from build123d import *

# Parameters (mm, degrees)
F1_DEPTH = 12.7
F3_DEPTH = 6.35
F4_R     = 2.54
F5_DEPTH = 12.7
F7_DEPTH = 76.201
F8_R     = 2.54
F9_DEPTH = 12.7


with BuildPart() as f1:
    # F0 (on Top) → F1 (new body)
    with BuildSketch(Plane.XY):
        Polygon((-68.2625, 38.1), (-68.2625, -38.1), (-55.5625, -38.1), (-55.5625, -25.4), (-4.7625, -12.7), (68.2625, -12.7), (68.2625, -5.08), (26.9875, -5.08), (26.9875, 5.08), (68.2625, 5.08), (68.2625, 12.7), (-4.7625, 12.7), (-55.5625, 25.4), (-55.5625, 38.1), align=None)
        Polygon((-49.2125, -12.7), (-49.2125, 12.7), (-18.1300211438, 6.223735015), (-18.1300211438, -6.223735015), align=None, mode=Mode.SUBTRACT)
    extrude(amount=F1_DEPTH)

    # F2 (on face) → F3 (cut)
    with BuildSketch(Plane.XY.offset(12.7)):
        Polygon((-55.5625, 25.4), (-55.5625, -25.4), (-4.7625, -12.7), (55.5625, -12.7), (55.5625, -5.08), (26.9875, -5.08), (26.9875, 5.08), (55.5625, 5.08), (55.5625, 12.7), (-4.7625, 12.7), align=None)
        Polygon((-49.2125, -12.7), (-49.2125, 12.7), (-18.1300211438, 6.223735015), (-18.1300211438, -6.223735015), align=None, mode=Mode.SUBTRACT)
    extrude(amount=-F3_DEPTH, mode=Mode.SUBTRACT)

    # F4 (on face) → F5 (cut)
    with BuildSketch(Plane.XZ.offset(38.1)):
        with Locations((-61.9125, 6.35)):
            Circle(F4_R)
    extrude(amount=-F5_DEPTH, mode=Mode.SUBTRACT)

    # F6 (on face) → F7 (cut, through all)
    with BuildSketch(Plane.XZ.offset(38.1)):
        with BuildLine():
            Line((61.9125, 6.35), (60.1164487758, 4.5539487758))
            ThreePointArc((60.1164487758, 4.5539487758), (61.9125, 3.81), (63.7085512242, 4.5539487758))
            Line((63.7085512242, 4.5539487758), (61.9125, 6.35))
        make_face()
        with BuildLine():
            Line((61.9125, 6.35), (60.1164487758, 8.1460512242))
            ThreePointArc((60.1164487758, 8.1460512242), (59.3725, 6.35), (60.1164487758, 4.5539487758))
            Line((60.1164487758, 4.5539487758), (61.9125, 6.35))
        make_face()
        with BuildLine():
            ThreePointArc((63.7085512242, 8.1460512242), (61.9125, 8.89), (60.1164487758, 8.1460512242))
            Line((60.1164487758, 8.1460512242), (61.9125, 6.35))
            Line((61.9125, 6.35), (63.7085512242, 8.1460512242))
        make_face()
        with BuildLine():
            ThreePointArc((64.4525, 6.35), (64.2591540126, 7.3220159182), (63.7085512242, 8.1460512242))
            Line((63.7085512242, 8.1460512242), (61.9125, 6.35))
            Line((61.9125, 6.35), (63.7085512242, 4.5539487758))
            ThreePointArc((63.7085512242, 4.5539487758), (64.2591540126, 5.3779840818), (64.4525, 6.35))
        make_face()
    extrude(amount=-F7_DEPTH, mode=Mode.SUBTRACT)

    # F8 (on face) → F9 (cut)
    with BuildSketch(Plane(origin=(0, 38.1, 0), x_dir=(-1, 0, 0), z_dir=(0, 1, 0))):
        with Locations((61.9125, 6.35)):
            Circle(F8_R)
    extrude(amount=-F9_DEPTH, mode=Mode.SUBTRACT)


solid = f1.part
Read the model definition and answer for the solid it produces. Units are mm, in the model's axes. A direction names the side the tool comes from. Coordinates: 2 decimals unless noted, no trailing zeros. Loops run counter-clockwise (first coordinate to the right, second up) from the corner with the lowest first, then second, coordinate; pieces in that order, holes last. Notation, with made-up numbers: (57.25, 59.25) -> (68.25, 59.25) arc R8 cw to (68.25, 71.25) -> close; hole circle Ø11 at (-1.75, 47.5). An arc over 180 degrees is marked (long way). Write item = value, one per line. Start each with the question number.
1) The part is cut by section A-A, the plane y = 8.5. Determine the outline of the cut face in (x, z).
2) Given P1, Ø3, axis at x = -61.91, z = 6.35, coming from the +Y side; P2, Ø3, axis at x = 45.5, z = 5, coming from the +Y side; P3, Ø3, axis at x = 46, y = 9, coming from the +Z side; P4, Ø4, axis at x = 41, y = -2, coming from the -Z side, each flat-ended and moving along its own axis, determine where each tip first touches the part or whether it passes through.
3) The mould has two halves that part along Z. Classify faces 5 (the face through (-65, -38.1, 6)), 6 (the face through (62, -9, 12.7)), 7 (the face through (-62, -25.4, 6)), 8 (the face through (-62, 25.4, 6)): pulls with the +Z half, pulls with the -Z half, needs draft (parallel to the pull), parting line crosses it, or undercut.
4) The part is cut by section D-D, the plane x = -33. Determine the outline of the cut face in (y, z).
5) Find the intervals of material crossed by L1, parallel to X at y = 11.5, z = 6.5; L2, parallel to X at y = -10, z = 9.25; L3, parallel to Y at x = 36, z = 2, in increasing order. Write a range as from..to.
6) For faces 1 (the face through (31, -12.7, 5)), 2 (the face through (-64.45, -31.84, 6.46)), 3 (the face through (-33.889, 9.507, 3.131)), 4 (the face through (52, 5.08, 5)), determine the directions among +Z, -Z, +X, -X, +Y, -Y from which every point of the face is accessible in a straight line to the end or side of a thin tool.
7) The part is cut by section C-C, the plane y = -3.5. Determine the outline of the cut face in (x, z).
8) The part is cut by section B-B, the plane x = 45.5. Determine the outline of the cut face in (y, z), plus the area to 3 significant figures.
Result:
q1.outline = (-68.26, 0) -> (-49.21, 0) -> (-49.21, 6.35) -> (-55.56, 6.35) -> (-55.56, 12.7) -> (-68.26, 12.7) -> close; (-29.05, 0) -> (68.26, 0) -> (68.26, 12.7) -> (55.56, 12.7) -> (55.56, 6.35) -> (-29.05, 6.35) -> close; hole circle Ø5.08 at (61.91, 6.35)
q2.P1 = 25.4
q2.P2 = 12.7
q2.P3 = 6.35
q2.P4 = through
q3.face_5 = needs draft
q3.face_6 = pulls with the +Z half
q3.face_7 = undercut
q3.face_8 = undercut
q4.outline = (-19.76, 0) -> (-9.32, 0) -> (-9.32, 6.35) -> (-19.76, 6.35) -> close; (9.32, 0) -> (19.76, 0) -> (19.76, 6.35) -> (9.32, 6.35) -> close
q5.L1 = -68.26..-55.56, 55.56..59.38, 64.45..68.26
q5.L2 = -68.26..-55.56, 55.56..68.26
q5.L3 = -12.7..-5.08, 5.08..12.7
q6.face_1 = +Z, -Z, +X, -Y
q6.face_2 = -Y
q6.face_3 = +Z, -Z
q6.face_4 = +Z, -Z, +X
q7.outline = (-68.26, 0) -> (-49.21, 0) -> (-49.21, 6.35) -> (-55.56, 6.35) -> (-55.56, 12.7) -> (-68.26, 12.7) -> close; (-18.13, 0) -> (26.99, 0) -> (26.99, 6.35) -> (-18.13, 6.35) -> close
q8.outline = (-12.7, 0) -> (-5.08, 0) -> (-5.08, 6.35) -> (-12.7, 6.35) -> close; (5.08, 0) -> (12.7, 0) -> (12.7, 6.35) -> (5.08, 6.35) -> close
q8.area = 96.8 mm²
